Geometry: see drawing. Coordinates: mm, zero at the bounding-box minimum. Coordinates: 2 decimals unless noted, no trailing zeros. Order: outer loops, then holes, each group sorted by start corner. A loop starts at its lowest first (then second) coordinate and runs counter-clockwise, first axis right, second up.
Item 1: Section C-C on x = 11.25. Return the cut outline in (y, z), then the cut area to 3 significant figures.
Item 2: Ray query, line 1 (Y direction, x = 10.5, z = 1.25); line 2 (Y direction, x = 11, z = 0.6); line 3 (X direction, y = 25.5, z = 1.75). Return the intervals inside material, ascending.
Item 3: Contact query for flat-ended pins moving along their axis: P1, Ø8, axis at x = 9.525, y = 45.8, coming from the -Z side; P2, Ø6, axis at x = 10, y = 25, coming from the +Z side. Output: stop coordinate, or through.
Item 4: Section B-B on x = 3.75. Return the cut outline in (y, z), then the cut area to 3 significant figures.
Item 5: Section D-D on z = 0.9. Return the cut outline in (x, y) (3 decimals).
Item 6: Section A-A on y = 25.4. Return the cut outline in (x, z) (3 decimals).
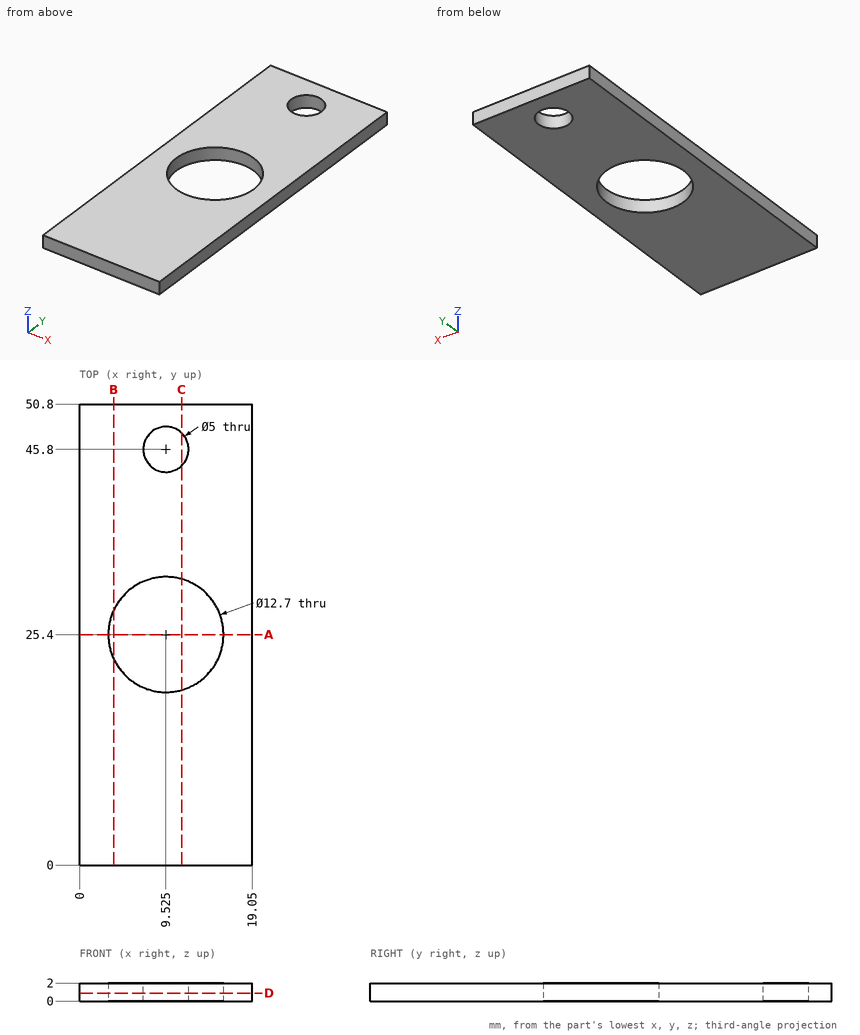
Answer list:
1. outline: (0, 0) - (19.29, 0) - (19.29, 2) - (0, 2) - close; (31.51, 0) - (43.99, 0) - (43.99, 2) - (31.51, 2) - close; (47.61, 0) - (50.8, 0) - (50.8, 2) - (47.61, 2) - close
1. area: 69.9 mm2
2. line 1: y = 0 to 19.13, 31.67 to 43.5, 48.1 to 50.8
2. line 2: y = 0 to 19.22, 31.58 to 43.78, 47.82 to 50.8
2. line 3: x = 0 to 3.18, 15.87 to 19.05
3. P1: stops at z = 0
3. P2: passes through
4. outline: (0, 0) - (22.76, 0) - (22.76, 2) - (0, 2) - close; (28.04, 0) - (50.8, 0) - (50.8, 2) - (28.04, 2) - close
4. area: 91.0 mm2
5. outline: (0, 0) - (19.05, 0) - (19.05, 50.8) - (0, 50.8) - close; hole circle Ø12.7 at (9.525, 25.4); hole circle Ø5 at (9.525, 45.8)
6. outline: (0, 0) - (3.175, 0) - (3.175, 2) - (0, 2) - close; (15.875, 0) - (19.05, 0) - (19.05, 2) - (15.875, 2) - close
